For this review, take the finished solid that the model builds, in its own axes (mm). Face numbers are marked on the shaded views. A direction names the side the tool comes from. Give positions to 0.01 mm unless a question says otherwise; leave off trailing zeros. Write each loop counter-clockwise with the first axis right and the second up, starting at its lowest first coordinate (ties: lowest second). Pieces come first, ordered by that corner, then holes.
Q1. We need section A-A (x = -17). Write out the cut boundary in (y, z).
Q2. Mouldability with a two-part tool opening along Y and no side actions: class the marked faces 1, 2, 3 and 4 as released by +Y, released by -Y, zero draft, split by the parting line, or undercut.
Q3. We need section B-B (z = -12). Write out the cut boundary in (x, y).
Q4. For line 1 (Y direction, x = 140, z = -8.5); line 2 (Y direction, x = 0, z = -8.25); line 3 (X direction, y = -3, z = -4), list the stretches that pass through material, from the lowest coordinate up.
Q5. We need section D-D (x = 52.5). Write out the cut boundary in (y, z), then the cut area to 3 significant figures.
Q6. We need section C-C (y = 23). Write out the cut boundary in (x, z).
Q7. Machinability: for the marked faces 5, 6 and 7, which of the approach directions +Z, -Z, +X, -X, +Y, -Y give a long, thin tool a straight path to every point of the face, cutting with its end or side? Answer none if there is none.
Q8. Insertion check: P1, Ø6, axis at y = 29, z = -12, coming from the +X side; P2, Ø18, axis at x = 69.5, y = 4, coming from the -Z side; P3, Ø1.5, axis at x = -4, z = -7, coming from the -Y side; P4, Ø10, axis at x = 62, y = -27.5, coming from the -Z side. Each pin has a flat end and moves straight along its axis. Give the tip position at first contact, or say it passes through.
```python
from build123d import *

# Parameters (mm, degrees)
SKETCH1_R          = 30
SKETCH1_R_2        = 7
BASE_EXTRUDE_DEPTH = 20
FILLET1_R          = 10
FILLET2_R          = 20
CUT_EXTRUDE1_DEPTH = 5
CUT_EXTRUDE2_DEPTH = 5


with BuildPart() as part:
    # Sketch1 → Base-Extrude (new body)
    with BuildSketch(Plane.XY):
        with BuildLine():
            Line((27.935473676, 25.760615491), (128.063755469, 9.084385863))
            ThreePointArc((128.063755469, 9.084385863), (155, 0), (128.063755469, -9.084385863))
            Line((128.063755469, -9.084385863), (27.935473676, -25.760615491))
            ThreePointArc((27.935473676, -25.760615491), (-38, 0), (27.935473676, 25.760615491))
        make_face()
        Circle(SKETCH1_R, mode=Mode.SUBTRACT)
        with Locations((140, 0)):
            Circle(SKETCH1_R_2, mode=Mode.SUBTRACT)
    extrude(amount=-BASE_EXTRUDE_DEPTH)

    # Fillet1
    fillet1_edges = [part.edges().sort_by_distance(p)[0] for p in [
        (128.063755469, 9.084385863, -10),
        (128.063755469, -9.084385863, -10),
    ]]
    fillet(fillet1_edges, radius=FILLET1_R)

    # Fillet2
    fillet2_edges = [part.edges().sort_by_distance(p)[0] for p in [
        (27.935473676, 25.760615491, -10),
        (27.935473676, -25.760615491, -10),
    ]]
    fillet(fillet2_edges, radius=FILLET2_R)

    # Sketch2 → Cut-Extrude1 (cut)
    with BuildSketch(Plane.XY):
        with BuildLine():
            Line((41.828554558, 17.870982725), (121.046940728, 4.677267873))
            ThreePointArc((121.046940728, 4.677267873), (123.741079282, 3.147292859), (124.807655013, 0.238406077))
            ThreePointArc((124.807655013, 0.238406077), (123.914202634, -2.958553332), (121.071833732, -4.673121977))
            Line((121.071833732, -4.673121977), (41.828554558, -17.870982725))
            ThreePointArc((41.828554558, -17.870982725), (37.231968897, -16.217361812), (36.238855523, -11.43439331))
            ThreePointArc((36.238855523, -11.43439331), (38, 0), (36.238855523, 11.43439331))
            ThreePointArc((36.238855523, 11.43439331), (37.231968897, 16.217361812), (41.828554558, 17.870982725))
        make_face()
    extrude(amount=-CUT_EXTRUDE1_DEPTH, mode=Mode.SUBTRACT)

    # Sketch3 → Cut-Extrude2 (cut)
    with BuildSketch(Plane(origin=(0, 0, -20), x_dir=(-1, 0, 0), z_dir=(0, 0, -1))):
        with BuildLine():
            Line((-121.445609231, 4.610870174), (-41.828554558, 17.870982725))
            ThreePointArc((-41.828554558, 17.870982725), (-37.231968897, 16.217361812), (-36.238855523, 11.43439331))
            ThreePointArc((-36.238855523, 11.43439331), (-38, 0), (-36.238855523, -11.43439331))
            ThreePointArc((-36.238855523, -11.43439331), (-37.231968897, -16.217361812), (-41.828554558, -17.870982725))
            Line((-41.828554558, -17.870982725), (-121.433526351, -4.612882562))
            ThreePointArc((-121.433526351, -4.612882562), (-124.132861899, -3.076762276), (-125.194211834, -0.157924451))
            ThreePointArc((-125.194211834, -0.157924451), (-124.244145959, 2.952985869), (-121.445609231, 4.610870174))
        make_face()
    extrude(amount=-CUT_EXTRUDE2_DEPTH, mode=Mode.SUBTRACT)


solid = part.part
```
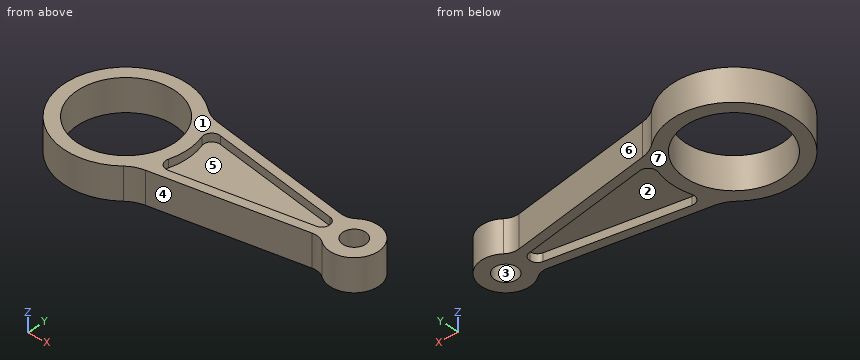
Computed:
1. outline: (-33.99, -20) - (-24.72, -20) - (-24.72, 0) - (-33.99, 0) - close; (24.72, -20) - (33.99, -20) - (33.99, 0) - (24.72, 0) - close
2. face 1: zero draft
2. face 2: undercut
2. face 3: undercut
2. face 4: released by -Y
3. outline: (24.38, -29.15) arc R20 cw to (33.92, -24.76) - (123.07, -9.92) arc R10 cw to (130.83, -11.87) arc R15 ccw (long way) to (130.83, 11.87) arc R10 cw to (123.07, 9.92) - (33.92, 24.76) arc R20 cw to (24.38, 29.15) arc R38 ccw (long way) to start; hole circle Ø60 at (0, 0); hole circle Ø14 at (140, 0)
4. line 1: y = -15 to -7, 7 to 15
4. line 2: y = -38 to -30, 30 to 38
4. line 3: x = -37.88 to -29.85, 29.85 to 37.88, 123.88 to 133.68, 146.32 to 154.7
5. outline: (-21.67, -20) - (-16.09, -20) - (-16.09, -15) - (16.09, -15) - (16.09, -20) - (21.67, -20) - (21.67, 0) - (16.09, 0) - (16.09, -5) - (-16.09, -5) - (-16.09, 0) - (-21.67, 0) - close
5. area: 545 mm2
6. outline: (-30.25, -20) - (-19.26, -20) - (-19.26, 0) - (-30.25, 0) - close; (19.26, -20) - (44.51, -20) - (44.51, 0) - (19.26, 0) - close
7. face 5: +Z
7. face 6: +Z, -Z, +Y
7. face 7: -Z, +X, -X, +Y, -Y
8. P1: stops at x = 29.59
8. P2: stops at z = -15
8. P3: stops at y = -37.86
8. P4: passes through
